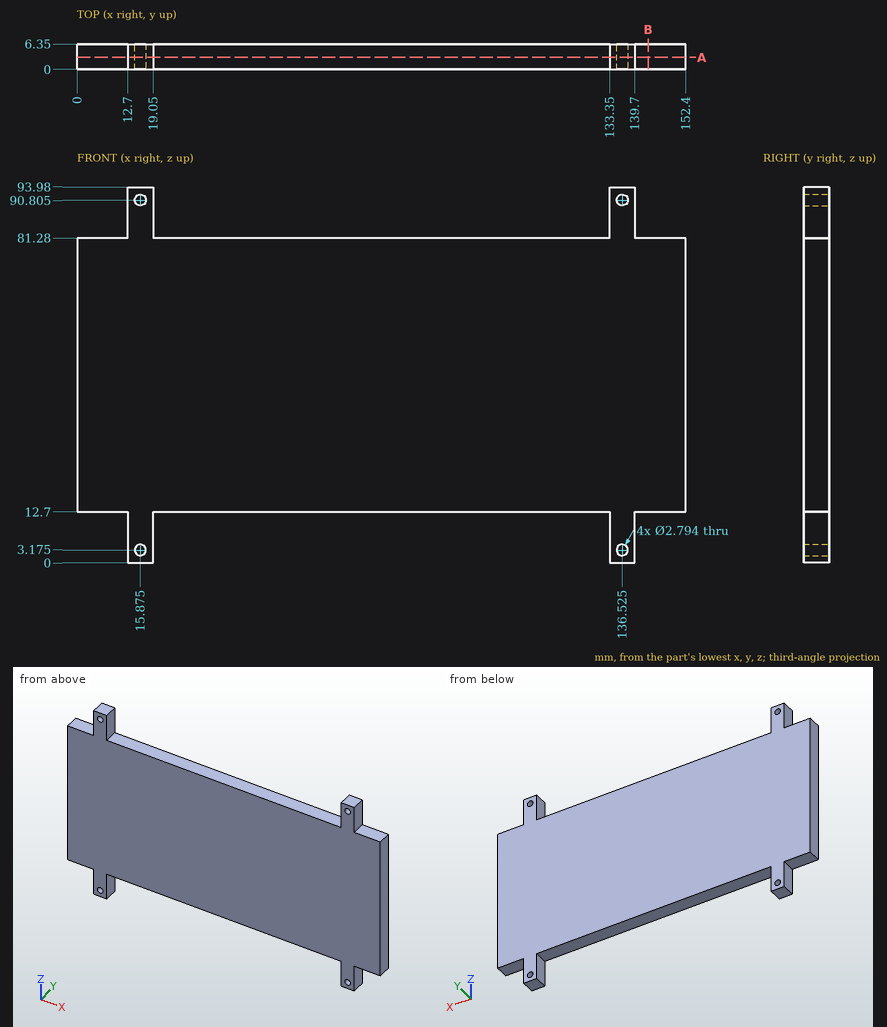
For this review, use the dimensioned drawing (mm, ordinates from the lowest corner) and the shaded views. Round coordinates to 2 decimals unless told otherwise and drop trailing zeros. Order: outer loops, then holes, each group sorted by start corner. A loop starts at its lowest first (then second) coordinate and runs counter-clockwise, first axis right, second up. Notation, with made-up numbers: (-6.5, 68.5) -> (21.5, 68.5) arc R24 cw to (21.5, 99.5) -> close; hole circle Ø8 at (83.5, 5.5). An arc over 180 degrees is marked (long way). Put each result on its own line as item: value.
Q1. Add section B-B on x = 143. Write out the cut boundary in (y, z).
Check result:
outline: (0, 12.7) -> (6.35, 12.7) -> (6.35, 81.28) -> (0, 81.28) -> close
Q2. For probe 1 along X at (y, z) = (1.5, 11.5); probe 2 along Z at (x, y) = (137.5, 3.25); probe 3 along Z at (x, y) = (103, 4.5), list the stretches that pass through material, from the lowest coordinate up. Write a range as [from, to].
Check result:
probe 1: [12.7, 19.05], [133.35, 139.7]
probe 2: [0, 2.17], [4.18, 89.8], [91.81, 93.98]
probe 3: [12.7, 81.28]
Q3. Insertion check: pin 1 Ø1 at (y, z) = (5.5, 83) entering from -X; pin 2 Ø1.5 at (x, y) = (118, 4.5) entering from -Z; pin 3 Ø3 at (y, z) = (2, 89) entering from +X; pin 4 Ø2.5 at (x, z) = (15.875, 3.175) entering from -Y. Each pin has a flat end and moves straight along its axis. Give the tip position at first contact, or say it passes through.
Check result:
pin 1: x = 12.7
pin 2: z = 12.7
pin 3: x = 139.7
pin 4: through
Q4. Add section A-A on y = 3. Write out the cut boundary in (x, z) (3 decimals), plus the area to 3 significant figures.
Check result:
outline: (0, 12.7) -> (12.7, 12.7) -> (12.7, 0) -> (19.05, 0) -> (19.05, 12.7) -> (133.35, 12.7) -> (133.35, 0) -> (139.7, 0) -> (139.7, 12.7) -> (152.4, 12.7) -> (152.4, 81.28) -> (139.7, 81.28) -> (139.7, 93.98) -> (133.35, 93.98) -> (133.35, 81.28) -> (19.05, 81.28) -> (19.05, 93.98) -> (12.7, 93.98) -> (12.7, 81.28) -> (0, 81.28) -> close; hole circle Ø2.794 at (15.875, 3.175); hole circle Ø2.794 at (15.875, 90.805); hole circle Ø2.794 at (136.525, 3.175); hole circle Ø2.794 at (136.525, 90.805)
area: 10,700 mm2
